The listing builds one solid part. Answer for the finished solid, in the listing's coordinates (mm). A direction names the side the tool comes from. Coordinates: 2 decimals unless noted, no trailing zeros. Order: outer loops, then holes, each group sorted by start corner. A loop starts at its lowest first (then second) coordinate and runs counter-clockwise, first axis right, second up. Notation, with made-up numbers: (86.5, 46.25) -> (112.5, 46.25) arc R25 ccw to (112.5, 69.25) -> close; hole circle Ø6 at (15.25, 25). An arc over 180 degrees is marked (long way). Return JSON: item names as keys, results as strings.
from build123d import *

# Parameters (mm, degrees)
SKETCH_1_R = 7
SKETCH_3_R = 6


with BuildPart() as part:
    # Sweep 1: sweep along a path in 草图2
    with BuildLine(Plane(origin=(0, 0, 0), x_dir=(0, 0, -1), z_dir=(1, 0, 0))) as sweep_1_path:
        Line((0, 0), (10, 0))
        ThreePointArc((10, 0), (17.071067812, -2.928932188), (20, -10))
        Line((20, -10), (20, -20))
    # 草图1 → Sweep 1 (sweep)
    with BuildSketch(Plane.XY):
        Circle(SKETCH_1_R)
    sweep(path=sweep_1_path.line)

    # Sweep 1 2: sweep along a path in 草图4
    with BuildLine(Plane(origin=(0, 0, 0), x_dir=(0, 0, -1), z_dir=(1, 0, 0))) as sweep_1_2_path:
        Line((0, 0), (10, 0))
        ThreePointArc((10, 0), (17.071067812, -2.928932188), (20, -10))
        Line((20, -10), (20, -20))
    # 草图3 → Sweep 1 2 (sweep, cut)
    with BuildSketch(Plane.XY):
        Circle(SKETCH_3_R)
    sweep(path=sweep_1_2_path.line, mode=Mode.SUBTRACT)


solid = part.part
1. The part is cut by section B-B on z = -3.25. Give the vertices of the cut face in (x, y), and give its area (3 significant figures).
Answer block:
{"outline": "circle Ø14 at (0, 0); hole circle Ø12 at (0, 0)", "area": "40.8 mm2"}
2. For faces 1 (the face through (-1.517, -15.07, -26.834)), 2 (the face through (-6, 0, -5)), 3 (the face through (2, -20, -14)), determine the directions among +Z, -Z, +X, -X, +Y, -Y from which every point of the face is accessible in a straight line to the end or side of a thin tool.
Answer block:
{"face 1": "-Y", "face 2": "+Z", "face 3": "+Z, -Z, +X, -X, -Y"}
3. Consider line 1 (Z direction, x = -0.25, y = -19); line 2 (Y direction, x = 0, z = -2.5). Determine where each line is inside the solid, lowest interval first. Write a range as from..to.
Answer block:
{"line 1": "z = -27..-25.99, -14.01..-13", "line 2": "y = -7..-6, 6..7"}
4. The part is cut by section A-A on x = 0. Give the vertices of the cut face in (y, z), and give its area (3 significant figures).
Answer block:
{"outline": "(-20, -27) -> (-10, -27) arc R17 ccw to (7, -10) -> (7, 0) -> (6, 0) -> (6, -10) arc R16 cw to (-10, -26) -> (-20, -26) -> close; (-20, -14) -> (-10, -14) arc R4 ccw to (-6, -10) -> (-6, 0) -> (-7, 0) -> (-7, -10) arc R3 cw to (-10, -13) -> (-20, -13) -> close", "area": "71.4 mm2"}
5. Each of these flat-tipped pins is pushed along its axis until it touches: pin 1 Ø1.5 at (x, z) = (-2, -9) entering from -Y; pin 2 Ø4 at (x, z) = (3, -13) entering from +Y; pin 3 Ø6 at (x, z) = (1.5, -20) entering from +Y. Where does it stop, or does it pass through?
Answer block:
{"pin 1": "stops at y = -6.89", "pin 2": "stops at y = 6.77", "pin 3": "stops at y = 5.4"}
6. The part is cut by section D-D on x = 3. Give the vertices of the cut face in (y, z), and give its area (3 significant figures).
Answer block:
{"outline": "(-20, -26.32) -> (-10, -26.32) arc R16.32 ccw to (6.32, -10) -> (6.32, 0) -> (5.2, 0) -> (5.2, -10) arc R15.2 cw to (-10, -25.2) -> (-20, -25.2) -> close; (-20, -14.8) -> (-10, -14.8) arc R4.8 ccw to (-5.2, -10) -> (-5.2, 0) -> (-6.32, 0) -> (-6.32, -10) arc R3.68 cw to (-10, -13.68) -> (-20, -13.68) -> close", "area": "80.6 mm2"}
7. The part is cut by section C-C on y = -15.25. Give the vertices of the cut face in (x, z), and give its area (3 significant figures).
Answer block:
{"outline": "circle Ø14 at (0, -20); hole circle Ø12 at (0, -20)", "area": "40.8 mm2"}
8. Determine the mould class of faces 4 (the face through (6.466, 2.681, -5.07)), 5 (the face through (-0.78, -15.07, -14.05)), 6 (the face through (6, 2, 0)) for opening direction X: pulls with the +X half, pulls with the -X half, needs draft (parallel to the pull), parting line crosses it, or undercut.
Answer block:
{"face 4": "parting line crosses it", "face 5": "undercut", "face 6": "needs draft"}
